Input: part model. Units: mm. Frame: model coordinates. A direction names the side the tool comes from. Round coordinates to 2 decimals unless told otherwise and drop trailing zeros. Order: outer loops, then holes, each group sorted by start corner. A loop starts at its lowest first (then second) coordinate and runs counter-clockwise, first axis right, second up.
Item 1: Reachability of faces 1 (the flat face through (0, 3, -60)), 2 (the flat face through (8.5, 2, 1)) from +Z, -Z, +X, -X, +Y, -Y: full face, straight path, thin tool, end or side. Return the list, or none.
Item 2: Mould query, pull axis Z, two halves, no side actions, for faces 3 (the flat face through (0, 0, -1)), 4 (the flat face through (0, 2, -68.5)), 5 (the flat face through (0, 3, 59)). Classes: released by +Z, released by -Z, zero draft, split by the parting line, or undercut.
Item 3: First-contact query: pin 1 (4 mm diameter, centred on x = 1, z = 59.5, fed in from +Y). Flat tip, straight axial feed; report the tip coordinate or a pass-through.
Item 4: Line query: L1, parallel to Y at x = 3.5, z = -57.5. Output: solid intervals per line, ascending.
Item 5: Cut plane B-B on z = -11.5. Output: boundary loops of the cut face in (x, y), then the cut area to 3 significant figures.
Item 6: Cut plane A-A on y = 4.25. Give the number of separate pieces and of enclosed holes in the cut face, then the cut area to 3 significant figures.
```python
from build123d import *

# Parameters (mm, degrees)
SKETCH1_W           = 17
SKETCH1_H           = 137
BOSS_EXTRUDE1_DEPTH = 5
SKETCH2_W           = 17
SKETCH2_H           = 13
CUT_EXTRUDE1_DEPTH  = 2
LPATTERN1_COUNT     = 8
LPATTERN1_PITCH     = 17


with BuildPart() as part:
    # Sketch1 → Boss-Extrude1 (new body)
    with BuildSketch(Plane(origin=(0, 0, 0), x_dir=(1, 0, 0), z_dir=(0, 1, 0))):
        Rectangle(SKETCH1_W, SKETCH1_H)
    extrude(amount=BOSS_EXTRUDE1_DEPTH)

    # Sketch2 → Cut-Extrude1 (cut)
    with BuildSketch(Plane(origin=(0, 5, 0), x_dir=(1, 0, 0), z_dir=(0, 1, 0))):
        with Locations((0, 59.5)):
            Rectangle(SKETCH2_W, SKETCH2_H)
    cut_extrude1 = extrude(amount=-CUT_EXTRUDE1_DEPTH, mode=Mode.SUBTRACT)

    # LPattern1: Cut-Extrude1 ×8
    with Locations(*[(0, 0, i * LPATTERN1_PITCH) for i in range(1, LPATTERN1_COUNT)]):
        add(cut_extrude1, mode=Mode.SUBTRACT)


solid = part.part
```
From the geometry:
1. face 1: +X, -X, +Y
1. face 2: +Z, -Z, +X, +Y, -Y
2. face 3: zero draft
2. face 4: released by -Z
2. face 5: undercut
3. pin 1: stops at y = 3
4. L1: y = 0 to 3
5. outline: (-8.5, 0) - (8.5, 0) - (8.5, 3) - (-8.5, 3) - close
5. area: 51.0 mm2
6. separate pieces: 9
6. enclosed holes: 0
6. area: 561 mm2
